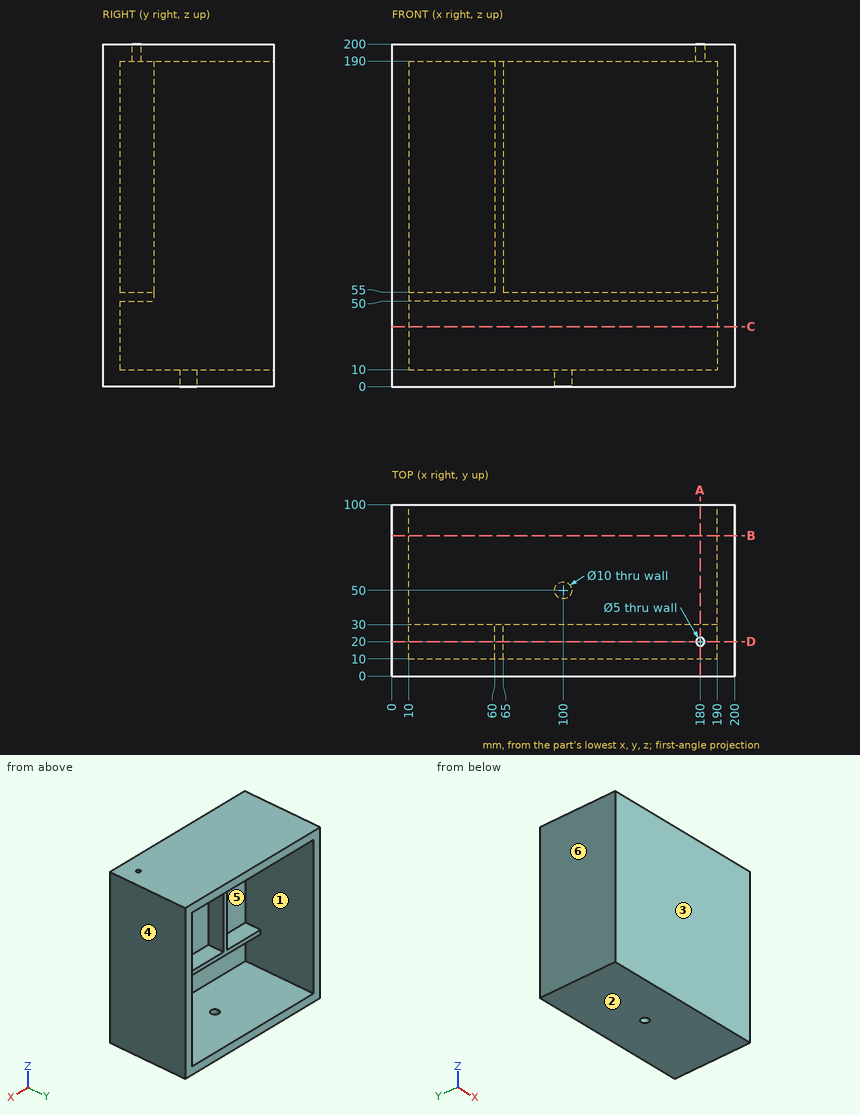
Study the drawing (mm; zero at the part's minimum x, y, z) and answer. A direction names the side the tool comes from. Round coordinates to 2 decimals unless told otherwise and drop trailing zeros. Write each loop counter-clockwise with the first axis right and the second up, starting at its lowest first coordinate (ties: lowest second). Pieces come first, ordered by that corner, then holes.
Q1. A tool of negligible diameter and unlimited length cuts with its end or side. For the marked faces 1 and 2, from which of +Z, -Z, +X, -X, +Y, -Y can it reach the whole face along a straight path? Write none if from no direction.
Values:
face 1: +Y
face 2: -Z, +X, -X, +Y, -Y
Q2. Find section A-A on x = 180. Determine the outline of the cut face in (y, z).
Values:
outline: (0, 0) - (100, 0) - (100, 10) - (10, 10) - (10, 50) - (30, 50) - (30, 55) - (10, 55) - (10, 190) - (17.5, 190) - (17.5, 200) - (0, 200) - close; (22.5, 190) - (100, 190) - (100, 200) - (22.5, 200) - close
Q3. Straight lines are drawn through the part: line 1 (Z direction, x = 31, y = 17); line 2 (X direction, y = 27, z = 107); line 3 (X direction, y = 77, z = 73). For each, find the intervals that lie inside material, in ascending order.
Values:
line 1: z = 0 to 10, 50 to 55, 190 to 200
line 2: x = 0 to 10, 60 to 65, 190 to 200
line 3: x = 0 to 10, 190 to 200
Q4. Find section C-C on z = 35. Determine the outline of the cut face in (x, y), and give its area (3 significant figures).
Values:
outline: (0, 0) - (200, 0) - (200, 100) - (190, 100) - (190, 10) - (10, 10) - (10, 100) - (0, 100) - close
area: 3,800 mm2
Q5. Find section B-B on y = 82. Determine the outline of the cut face in (x, z), and give its area (3 significant figures).
Values:
outline: (0, 0) - (200, 0) - (200, 200) - (0, 200) - close; hole (10, 10) - (190, 10) - (190, 190) - (10, 190) - close
area: 7,600 mm2
Q6. A flat-ended cylindrical pin translates along its axis: P1, Ø25, axis at x = 28, z = 113, coming from the +Y side. Find the tip coordinate at first contact, or state that the pin passes through.
Values:
P1: stops at y = 10
Q7. Find section D-D on y = 20. Determine the outline of the cut face in (x, z), and give its area (4 significant figures).
Values:
outline: (0, 0) - (200, 0) - (200, 200) - (182.5, 200) - (182.5, 190) - (190, 190) - (190, 55) - (65, 55) - (65, 190) - (177.5, 190) - (177.5, 200) - (0, 200) - close; hole (10, 10) - (190, 10) - (190, 50) - (10, 50) - close; hole (10, 55) - (60, 55) - (60, 190) - (10, 190) - close
area: 9,125 mm2
Q8. The mould has two halves that part along X. Classify the marked faces 3, 4, 5 and 6: released by +X, released by -X, zero draft, split by the parting line, or undercut.
Values:
face 3: zero draft
face 4: released by +X
face 5: undercut
face 6: released by -X
